from build123d import *

# Parameters (mm, degrees)
F0_R     = 9
F1_DEPTH = 1
F3_R     = 11
F4_DEPTH = 4
F6_R     = 14
F7_DEPTH = 1


with BuildPart() as f1:
    # F0 (on Top) → F1 (new body)
    with BuildSketch(Plane.XY):
        Circle(F0_R)
    extrude(amount=F1_DEPTH)

    # F3 (on offset) → F4 (join)
    with BuildSketch(Plane.XY.offset(1)):
        Circle(F3_R)
    extrude(amount=F4_DEPTH)

    # F6 (on offset) → F7 (join)
    with BuildSketch(Plane.XY.offset(5)):
        Circle(F6_R)
        with BuildLine():
            ThreePointArc((12.91588, 1.476495), (12.978953, 0.739444), (13, 0))
            ThreePointArc((13, 0), (12.978953, -0.739444), (12.91588, -1.476495))
            Line((12.91588, -1.476495), (13.642398, -1.642317))
            Line((13.642398, -1.642317), (13.003951, -4.439538))
            Line((13.003951, -4.439538), (12.277433, -4.273715))
            ThreePointArc((12.277433, -4.273715), (11.712595, -5.640489), (10.996179, -6.934266))
            Line((10.996179, -6.934266), (11.578801, -7.398892))
            Line((11.578801, -7.398892), (9.789912, -9.642088))
            Line((9.789912, -9.642088), (9.20729, -9.177463))
            ThreePointArc((9.20729, -9.177463), (8.105367, -10.163809), (6.89855, -11.018621))
            Line((6.89855, -11.018621), (7.221881, -11.690024))
            Line((7.221881, -11.690024), (4.63686, -12.934905))
            Line((4.63686, -12.934905), (4.31353, -12.263501))
            ThreePointArc((4.31353, -12.263501), (2.892772, -12.674063), (1.434578, -12.920603))
            Line((1.434578, -12.920603), (1.434578, -13.665805))
            Line((1.434578, -13.665805), (-1.434578, -13.665805))
            Line((-1.434578, -13.665805), (-1.434578, -12.920603))
            ThreePointArc((-1.434578, -12.920603), (-2.892772, -12.674063), (-4.31353, -12.263501))
            Line((-4.31353, -12.263501), (-4.63686, -12.934905))
            Line((-4.63686, -12.934905), (-7.221881, -11.690024))
            Line((-7.221881, -11.690024), (-6.89855, -11.018621))
            ThreePointArc((-6.89855, -11.018621), (-8.105367, -10.163809), (-9.20729, -9.177463))
            Line((-9.20729, -9.177463), (-9.789912, -9.642088))
            Line((-9.789912, -9.642088), (-11.578801, -7.398892))
            Line((-11.578801, -7.398892), (-10.996179, -6.934266))
            ThreePointArc((-10.996179, -6.934266), (-11.712595, -5.640489), (-12.277433, -4.273715))
            Line((-12.277433, -4.273715), (-13.003951, -4.439538))
            Line((-13.003951, -4.439538), (-13.642398, -1.642317))
            Line((-13.642398, -1.642317), (-12.91588, -1.476495))
            ThreePointArc((-12.91588, -1.476495), (-13, 0), (-12.91588, 1.476495))
            Line((-12.91588, 1.476495), (-13.642398, 1.642317))
            Line((-13.642398, 1.642317), (-13.003951, 4.439538))
            Line((-13.003951, 4.439538), (-12.277433, 4.273715))
            ThreePointArc((-12.277433, 4.273715), (-11.712595, 5.640489), (-10.996179, 6.934266))
            Line((-10.996179, 6.934266), (-11.578801, 7.398892))
            Line((-11.578801, 7.398892), (-9.789912, 9.642088))
            Line((-9.789912, 9.642088), (-9.20729, 9.177463))
            ThreePointArc((-9.20729, 9.177463), (-8.105367, 10.163809), (-6.89855, 11.018621))
            Line((-6.89855, 11.018621), (-7.221881, 11.690024))
            Line((-7.221881, 11.690024), (-4.63686, 12.934905))
            Line((-4.63686, 12.934905), (-4.31353, 12.263501))
            ThreePointArc((-4.31353, 12.263501), (-2.892772, 12.674063), (-1.434578, 12.920603))
            Line((-1.434578, 12.920603), (-1.434578, 13.665805))
            Line((-1.434578, 13.665805), (1.434578, 13.665805))
            Line((1.434578, 13.665805), (1.434578, 12.920603))
            ThreePointArc((1.434578, 12.920603), (2.892772, 12.674063), (4.31353, 12.263501))
            Line((4.31353, 12.263501), (4.63686, 12.934905))
            Line((4.63686, 12.934905), (7.221881, 11.690024))
            Line((7.221881, 11.690024), (6.89855, 11.018621))
            ThreePointArc((6.89855, 11.018621), (8.105367, 10.163809), (9.20729, 9.177463))
            Line((9.20729, 9.177463), (9.789912, 9.642088))
            Line((9.789912, 9.642088), (11.578801, 7.398892))
            Line((11.578801, 7.398892), (10.996179, 6.934266))
            ThreePointArc((10.996179, 6.934266), (11.712595, 5.640489), (12.277433, 4.273715))
            Line((12.277433, 4.273715), (13.003951, 4.439538))
            Line((13.003951, 4.439538), (13.642398, 1.642317))
            Line((13.642398, 1.642317), (12.91588, 1.476495))
        make_face(mode=Mode.SUBTRACT)
        with BuildLine():
            ThreePointArc((12.91588, -1.476495), (12.978953, -0.739444), (13, 0))
            ThreePointArc((13, 0), (12.978953, 0.739444), (12.91588, 1.476495))
            Line((12.91588, 1.476495), (10.807824, 0.995345))
            Line((10.807824, 0.995345), (10.169377, 3.792565))
            Line((10.169377, 3.792565), (12.277433, 4.273715))
            ThreePointArc((12.277433, 4.273715), (11.712595, 5.640489), (10.996179, 6.934266))
            Line((10.996179, 6.934266), (9.30565, 5.586114))
            Line((9.30565, 5.586114), (7.51676, 7.82931))
            Line((7.51676, 7.82931), (9.20729, 9.177463))
            ThreePointArc((9.20729, 9.177463), (8.105367, 10.163809), (6.89855, 11.018621))
            Line((6.89855, 11.018621), (5.960377, 9.070485))
            Line((5.960377, 9.070485), (3.375356, 10.315365))
            Line((3.375356, 10.315365), (4.31353, 12.263501))
            ThreePointArc((4.31353, 12.263501), (2.892772, 12.674063), (1.434578, 12.920603))
            Line((1.434578, 12.920603), (1.434578, 10.758335))
            Line((1.434578, 10.758335), (-1.434578, 10.758335))
            Line((-1.434578, 10.758335), (-1.434578, 12.920603))
            ThreePointArc((-1.434578, 12.920603), (-2.892772, 12.674063), (-4.31353, 12.263501))
            Line((-4.31353, 12.263501), (-3.375356, 10.315365))
            Line((-3.375356, 10.315365), (-5.960377, 9.070485))
            Line((-5.960377, 9.070485), (-6.89855, 11.018621))
            ThreePointArc((-6.89855, 11.018621), (-8.105367, 10.163809), (-9.20729, 9.177463))
            Line((-9.20729, 9.177463), (-7.51676, 7.82931))
            Line((-7.51676, 7.82931), (-9.30565, 5.586114))
            Line((-9.30565, 5.586114), (-10.996179, 6.934266))
            ThreePointArc((-10.996179, 6.934266), (-11.712595, 5.640489), (-12.277433, 4.273715))
            Line((-12.277433, 4.273715), (-10.169377, 3.792565))
            Line((-10.169377, 3.792565), (-10.807824, 0.995345))
            Line((-10.807824, 0.995345), (-12.91588, 1.476495))
            ThreePointArc((-12.91588, 1.476495), (-13, 0), (-12.91588, -1.476495))
            Line((-12.91588, -1.476495), (-10.807824, -0.995345))
            Line((-10.807824, -0.995345), (-10.169377, -3.792565))
            Line((-10.169377, -3.792565), (-12.277433, -4.273715))
            ThreePointArc((-12.277433, -4.273715), (-11.712595, -5.640489), (-10.996179, -6.934266))
            Line((-10.996179, -6.934266), (-9.30565, -5.586114))
            Line((-9.30565, -5.586114), (-7.51676, -7.82931))
            Line((-7.51676, -7.82931), (-9.20729, -9.177463))
            ThreePointArc((-9.20729, -9.177463), (-8.105367, -10.163809), (-6.89855, -11.018621))
            Line((-6.89855, -11.018621), (-5.960377, -9.070485))
            Line((-5.960377, -9.070485), (-3.375356, -10.315365))
            Line((-3.375356, -10.315365), (-4.31353, -12.263501))
            ThreePointArc((-4.31353, -12.263501), (-2.892772, -12.674063), (-1.434578, -12.920603))
            Line((-1.434578, -12.920603), (-1.434578, -10.758335))
            Line((-1.434578, -10.758335), (1.434578, -10.758335))
            Line((1.434578, -10.758335), (1.434578, -12.920603))
            ThreePointArc((1.434578, -12.920603), (2.892772, -12.674063), (4.31353, -12.263501))
            Line((4.31353, -12.263501), (3.375356, -10.315365))
            Line((3.375356, -10.315365), (5.960377, -9.070485))
            Line((5.960377, -9.070485), (6.89855, -11.018621))
            ThreePointArc((6.89855, -11.018621), (8.105367, -10.163809), (9.20729, -9.177463))
            Line((9.20729, -9.177463), (7.51676, -7.82931))
            Line((7.51676, -7.82931), (9.30565, -5.586114))
            Line((9.30565, -5.586114), (10.996179, -6.934266))
            ThreePointArc((10.996179, -6.934266), (11.712595, -5.640489), (12.277433, -4.273715))
            Line((12.277433, -4.273715), (10.169377, -3.792565))
            Line((10.169377, -3.792565), (10.807824, -0.995345))
            Line((10.807824, -0.995345), (12.91588, -1.476495))
        make_face()
    extrude(amount=F7_DEPTH)


solid = f1.part
Could you check a few things on this model? Use its own coordinates, in mm. A direction names the side the tool comes from. Give positions to 0.01 mm unless a question says otherwise; leave off trailing zeros. Order: outer loops, then holes, each group sorted by start corner. A loop starts at its lowest first (then second) coordinate and runs counter-clockwise, first axis right, second up.
1. Suppose I cut it at A-A (x = 0). List the corners of the cut face in (y, z) for me.
2. Suppose I cut it at D-D (z = 3.3). List the corners of the cut face in (x, y) for me.
3. For faces 1 (the flat face through (0, 0, 6)), 2 (the flat face through (4.686, 9.684, 5.493)), 3 (the flat face through (-5.91, -12.32, 5.49)), which set-ups out of +Z, -Z, +X, -X, +Y, -Y let a thin tool reach every point of the face, with its end or its side?
4. I need wall thicknesses on L1, parallel to X at y = -3, z = 5.6; L2, parallel to X at y = 9, z = 5.25; L3, parallel to Z at x = 7.25, y = 10. Which ranges of each line are inside material? Lowest first, please.
5. We'd pull the mould along X, two halves only. Please class faces 4 (the flat face through (2, -9, 1)), 5 (the flat face through (10.493, 2.374, 5.493)): pulls with the +X half, pulls with the -X half, needs draft (parallel to the pull), parting line crosses it, or undercut.
6. Will these pins go through, and if not, where does the flat tip stop? P1, Ø3, axis at y = 10.5, z = 5, coming from the +X side; P2, Ø1.5, axis at x = -5, z = 5.5, coming from the -Y side; P3, Ø1, axis at x = -9, y = 7, coming from the +Z side.
7. Suppose I cut it at C-C (z = 5.6). Give the number of separate pieces and of enclosed holes in the cut face, plus the area to 3 significant figures.
8. Suppose I cut it at B-B (y = 2.75). List the corners of the cut face in (x, z) for me, plus the area to 3 significant figures.
Solved:
1. outline: (-14, 5) - (-13.67, 5) - (-13.67, 6) - (-14, 6) - close; (-11, 1) - (-9, 1) - (-9, 0) - (9, 0) - (9, 1) - (11, 1) - (11, 5) - (10.76, 5) - (10.76, 6) - (-10.76, 6) - (-10.76, 5) - (-11, 5) - close; (13.67, 5) - (14, 5) - (14, 6) - (13.67, 6) - close
2. outline: circle Ø22 at (0, 0)
3. face 1: +Z, +X, -X, +Y, -Y
3. face 2: +Z
3. face 3: +Z, -Z
4. L1: x = -13.67 to -13.33, -10.35 to 10.35, 13.33 to 13.67
4. L2: x = -10.72 to -10.3, -8.98 to 8.98, 10.3 to 10.72
4. L3: z = 5 to 6
5. face 4: needs draft
5. face 5: undercut
6. P1: stops at x = 10.72
6. P2: stops at y = -13.34
6. P3: stops at z = 5
7. separate pieces: 1
7. enclosed holes: 14
7. area: 499 mm2
8. outline: (-13.73, 5) - (-13.39, 5) - (-13.39, 6) - (-13.73, 6) - close; (-10.65, 1) - (-8.57, 1) - (-8.57, 0) - (8.57, 0) - (8.57, 1) - (10.65, 1) - (10.65, 5) - (10.41, 5) - (10.41, 6) - (-10.41, 6) - (-10.41, 5) - (-10.65, 5) - close; (13.39, 5) - (13.73, 5) - (13.73, 6) - (13.39, 6) - close
8. area: 124 mm2
